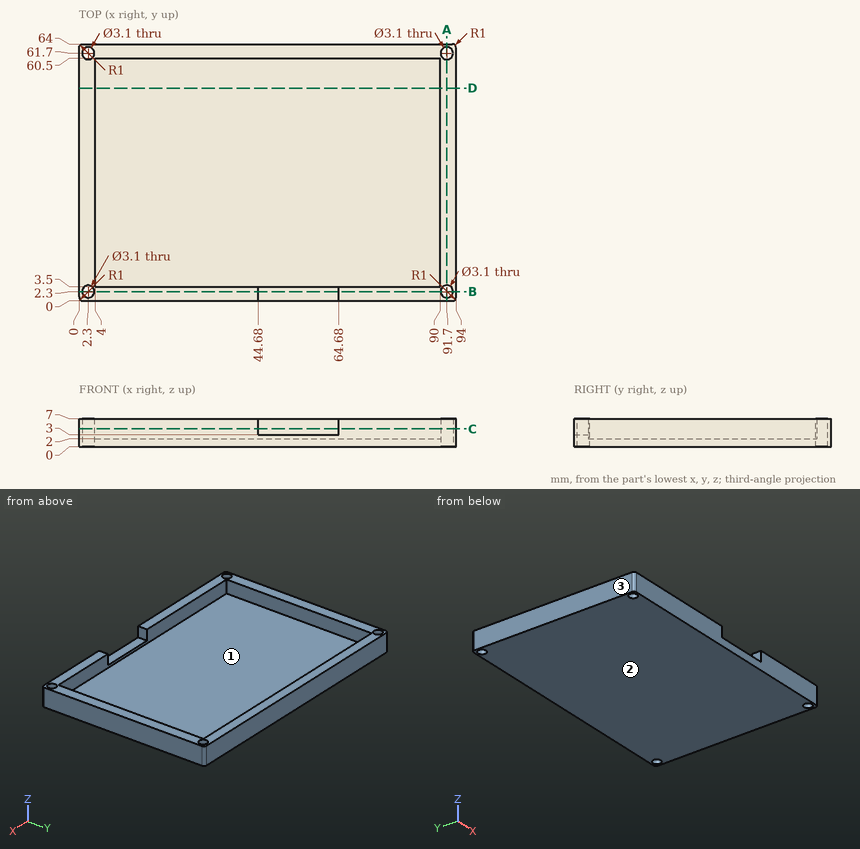
Part print with two shaded views. Sizes in mm from the minimum x, y, z corner. Round coordinates to 2 decimals unless told otherwise and drop trailing zeros. Order: outer loops, then holes, each group sorted by start corner. A loop starts at its lowest first (then second) coordinate and runs counter-clockwise, first axis right, second up. Notation, with made-up numbers: (82.5, -12.5) - (114.5, -12.5) arc R31 ccw to (114.5, 24.5) - close; hole circle Ø10 at (-40, 25.25). An arc over 180 degrees is marked (long way). Return JSON: item names as keys, results as strings.
(1) Cut at D-D (y = 53). Give the cut face in (x, z).
Answer key:
{"outline": "(0, 0) - (94, 0) - (94, 7) - (90, 7) - (90, 2) - (4, 2) - (4, 7) - (0, 7) - close"}
(2) Cut at C-C (z = 4.5). Give the cut face in (x, y).
Answer key:
{"outline": "(0, 1) arc R1 ccw to (1, 0) - (44.68, 0) - (44.68, 3.5) - (4, 3.5) - (4, 60.5) - (90, 60.5) - (90, 3.5) - (64.68, 3.5) - (64.68, 0) - (93, 0) arc R1 ccw to (94, 1) - (94, 63) arc R1 ccw to (93, 64) - (1, 64) arc R1 ccw to (0, 63) - close; hole circle Ø3.1 at (2.3, 2.3); hole circle Ø3.1 at (2.3, 61.7); hole circle Ø3.1 at (91.7, 2.3); hole circle Ø3.1 at (91.7, 61.7)"}
(3) Cut at A-A (x = 91.7). Give the cut face in (y, z), then the cut area to 3 significant figures.
Answer key:
{"outline": "(0, 0) - (0.75, 0) - (0.75, 7) - (0, 7) - close; (3.85, 0) - (60.15, 0) - (60.15, 7) - (3.85, 7) - close; (63.25, 0) - (64, 0) - (64, 7) - (63.25, 7) - close", "area": "405 mm^2"}
(4) Pin check, flat tips, straight feed: pin 1 Ø12 at (x, y) = (78, 49) entering from +Z; pin 2 Ø1.8 at (y, z) = (2.5, 4.5) entering from -X; pin 3 Ø1 at (x, y) = (54.5, 1) entering from +Z; pin 4 Ø3 at (x, y) = (91.7, 61.7) entering from +Z. Stop position of each tip, or through.
Answer key:
{"pin 1": "stops at z = 2", "pin 2": "stops at x = 0", "pin 3": "stops at z = 3", "pin 4": "passes through"}
(5) Pull direction X, two halves, no side cores. Call the marked faces 1, 2 and 3: +X half, -X half, draft (parallel to the pull), parting line (faces both ways), or undercut.
Answer key:
{"face 1": "undercut", "face 2": "draft", "face 3": "-X half"}
(6) Cut at B-B (y = 2.3). Give the cut face in (x, z).
Answer key:
{"outline": "(0, 0) - (0.75, 0) - (0.75, 7) - (0, 7) - close; (3.85, 0) - (90.15, 0) - (90.15, 7) - (64.68, 7) - (64.68, 3) - (44.68, 3) - (44.68, 7) - (3.85, 7) - close; (93.25, 0) - (94, 0) - (94, 7) - (93.25, 7) - close"}
(7) Wall check: probe 1 along X at (y, z) = (61.7, 2); probe 2 along Y at (x, z) = (91.7, 4); probe 3 along X at (y, z) = (21, 3.5). Give the ranges that are in metal, low to high. Write a range as from..to.
Answer key:
{"probe 1": "x = 0..0.75, 3.85..90.15, 93.25..94", "probe 2": "y = 0..0.75, 3.85..60.15, 63.25..64", "probe 3": "x = 0..4, 90..94"}
